Input: part model. Units: mm. Frame: model coordinates. Face numbers are marked on the shaded views. A direction names the side the tool comes from. Give positions to 0.01 mm unless a question says otherwise; leave off trailing zeros. Loops run counter-clockwise (first coordinate to the right, second up) from the corner with the lowest first, then second, coordinate; pieces in that order, holes last. Notation, with made-up numbers: (54.5, 83) -> (84.5, 83) arc R19 ccw to (84.5, 119) -> close; hole circle Ø9 at (71.5, 27.5). An arc over 180 degrees is marked (long way). Answer as a JSON object with one key per item and string values.
```python
from build123d import *

# Parameters (mm, degrees)
SKETCH1_W           = 55.5
SKETCH1_H           = 85.5
SKETCH1_W_2         = 53.5
SKETCH1_H_2         = 83.5
BOSS_EXTRUDE1_DEPTH = 54
SKETCH2_W           = 55.5
SKETCH2_H           = 85.5
BOSS_EXTRUDE2_DEPTH = 1
SKETCH3_W           = 11
SKETCH3_H           = 6
CUT_EXTRUDE1_DEPTH  = 1
SKETCH5_W           = 30
SKETCH5_H           = 5
BOSS_EXTRUDE4_DEPTH = 30
SKETCH8_W           = 16.2
SKETCH8_H           = 13
CUT_EXTRUDE3_DEPTH  = 1


with BuildPart() as part:
    # Sketch1 → Boss-Extrude1 (new body)
    with BuildSketch(Plane(origin=(0, 0, 0), x_dir=(1, 0, 0), z_dir=(0, 1, 0))):
        Rectangle(SKETCH1_W, SKETCH1_H)
        Rectangle(SKETCH1_W_2, SKETCH1_H_2, mode=Mode.SUBTRACT)
    extrude(amount=BOSS_EXTRUDE1_DEPTH)

    # Sketch2 → Boss-Extrude2 (add)
    with BuildSketch(Plane.XZ):
        Rectangle(SKETCH2_W, SKETCH2_H)
    extrude(amount=BOSS_EXTRUDE2_DEPTH)

    # Sketch3 → Cut-Extrude1 (cut)
    with BuildSketch(Plane.XY.offset(42.75)):
        with Locations((0, 14.9)):
            Rectangle(SKETCH3_W, SKETCH3_H)
    extrude(amount=-CUT_EXTRUDE1_DEPTH, mode=Mode.SUBTRACT)

    # Sketch5 → Boss-Extrude4 (add)
    with BuildSketch(Plane(origin=(0, 0, 41.75), x_dir=(-1, 0, 0), z_dir=(0, 0, -1))):
        with Locations((0.286122551, 23.4)):
            Rectangle(SKETCH5_W, SKETCH5_H)
    extrude(amount=BOSS_EXTRUDE4_DEPTH)

    # Sketch8 → Cut-Extrude3 (cut)
    with BuildSketch(Plane(origin=(0, 0, 41.75), x_dir=(-1, 0, 0), z_dir=(0, 0, -1))):
        with Locations((1.080339393, 46.6)):
            Rectangle(SKETCH8_W, SKETCH8_H)
    extrude(amount=-CUT_EXTRUDE3_DEPTH, mode=Mode.SUBTRACT)


solid = part.part
```
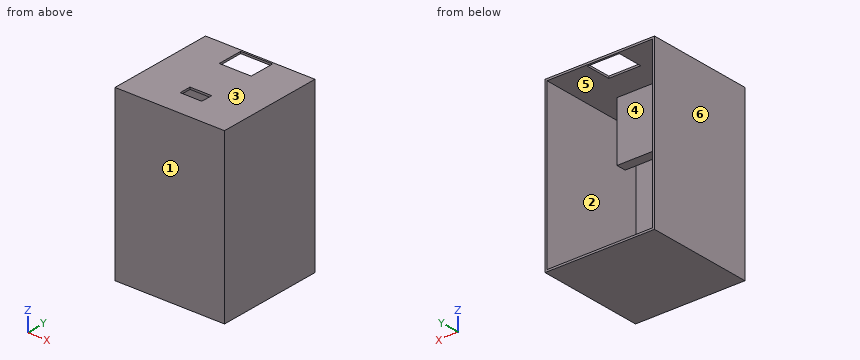
Q1. Section A-A, the plane x = -8. Return the cut outline in (y, z).
Evaluation:
{"outline": "(-1, -42.75) -> (54, -42.75) -> (54, -41.75) -> (0, -41.75) -> (0, 41.75) -> (20.9, 41.75) -> (20.9, 11.75) -> (25.9, 11.75) -> (25.9, 41.75) -> (40.1, 41.75) -> (40.1, 42.75) -> (-1, 42.75) -> close; (53.1, 41.75) -> (54, 41.75) -> (54, 42.75) -> (53.1, 42.75) -> close"}
Q2. Pin query (flat end, axial travel): pin 1 (4 mm diameter, centred on x = -12, z = -31, fed in from +Y). Return the tip coordinate at first contact, or that it passes through.
Evaluation:
{"pin 1": "stops at y = 0"}
Q3. Draft query along Z for the marked faces 1, 2, 3 and 4. Return one class per face: +Z half, -Z half, draft (parallel to the pull), parting line (faces both ways), or undercut.
Evaluation:
{"face 1": "draft", "face 2": "undercut", "face 3": "+Z half", "face 4": "undercut"}
Q4. Ray query, line 1 along X through (y, z) = (30, -26.5); line 2 along Z through (x, y) = (16.5, 2); line 3 along Y through (x, z) = (-9.5, 19.5). Return the intervals inside material, ascending.
Evaluation:
{"line 1": "x = -27.75 to -26.75, 26.75 to 27.75", "line 2": "z = -42.75 to -41.75, 41.75 to 42.75", "line 3": "y = -1 to 0, 20.9 to 25.9"}
Q5. Section B-B, the plane z = 33.5. Return the cut outline in (x, y).
Evaluation:
{"outline": "(-27.75, -1) -> (27.75, -1) -> (27.75, 54) -> (26.75, 54) -> (26.75, 0) -> (-26.75, 0) -> (-26.75, 54) -> (-27.75, 54) -> close; (-15.29, 20.9) -> (14.71, 20.9) -> (14.71, 25.9) -> (-15.29, 25.9) -> close"}
Q6. Section C-C, the plane y = 9.5. Return the cut outline in (x, z), then the cut area to 3 significant figures.
Evaluation:
{"outline": "(-27.75, -42.75) -> (27.75, -42.75) -> (27.75, 42.75) -> (-27.75, 42.75) -> close; hole (-26.75, -41.75) -> (26.75, -41.75) -> (26.75, 41.75) -> (-26.75, 41.75) -> close", "area": "278 mm2"}
Q7. Section D-D, the plane x = 19. Return the cut outline in (y, z).
Evaluation:
{"outline": "(-1, -42.75) -> (54, -42.75) -> (54, -41.75) -> (0, -41.75) -> (0, 41.75) -> (54, 41.75) -> (54, 42.75) -> (-1, 42.75) -> close"}
Q8. Access query for the marked faces 5 and 6. Directions: +Z, -Z, +X, -X, +Y, -Y. A direction counts if a zero-diameter tool reaches every point of the face in a straight line with its end or side. Return the directions, or none.
Evaluation:
{"face 5": "none", "face 6": "+Z, -Z, -X, +Y, -Y"}
